Check sheet for the modelled part. Datum: model origin and axes. Units: mm. A direction names the side the tool comes from. Coordinates: 2 decimals unless noted, no trailing zeros. Loops run counter-clockwise (first coordinate to the right, second up) from the corner with the lowest first, then second, coordinate; pieces in that order, holes last. Notation, with made-up numbers: (-23.5, 71) -> (34.5, 71) arc R25 cw to (34.5, 96) -> close; hole circle Ø7 at (-35, 41.25). An arc over 180 degrees is marked (long way). Use CSV: the item, a comma, the result in double quotes.
```python
from build123d import *

# Parameters (mm, degrees)
SKETCH1_W                      = 105
SKETCH1_H                      = 69
BOSS_EXTRUDE1_DEPTH            = 10
FILLET1_R                      = 3
CBORE_FOR_M3_SHCS1_D           = 3.4
CBORE_FOR_M3_SHCS1_CBORE_D     = 6.5
CBORE_FOR_M3_SHCS1_CBORE_DEPTH = 4


with BuildPart() as part:
    # Sketch1 → Boss-Extrude1 (new body)
    with BuildSketch(Plane(origin=(0, 0, 0), x_dir=(1, 0, 0), z_dir=(0, 1, 0))):
        Rectangle(SKETCH1_W, SKETCH1_H)
    extrude(amount=BOSS_EXTRUDE1_DEPTH)

    # Fillet1
    fillet1_edges = [part.edges().sort_by_distance(p)[0] for p in [
        (52.5, 5, 34.5),
        (-52.5, 5, 34.5),
        (-52.5, 5, -34.5),
        (52.5, 5, -34.5),
    ]]
    fillet(fillet1_edges, radius=FILLET1_R)

    # CBORE for M3 SHCS1 (through all)
    with Locations(Plane(origin=(0, 10, 0), x_dir=(1, 0, 0), z_dir=(0, 1, 0))):
        with Locations((0, 0)):
            CounterBoreHole(CBORE_FOR_M3_SHCS1_D / 2, CBORE_FOR_M3_SHCS1_CBORE_D / 2, CBORE_FOR_M3_SHCS1_CBORE_DEPTH)

    # Sketch5 → M3x0.5 Tapped Hole1 (revolve, cut)
    with BuildSketch(Plane(origin=(16.5, 10, 22), x_dir=(0, 0, 1), z_dir=(1, 0, 0))):
        Polygon((0, 0), (0, 10.751075774), (1.25, 10), (1.25, 0), align=None)
    m3x0_5_tapped_hole1 = revolve(axis=Axis((16.5, 16.35, 22), (0, -1, 0)), mode=Mode.SUBTRACT)

    # Mirror1: M3x0.5 Tapped Hole1 across plane
    add(m3x0_5_tapped_hole1.mirror(Plane(origin=(0, 0, 0), x_dir=(0, 0, 1), z_dir=(1, 0, 0))), mode=Mode.SUBTRACT)

    # Mirror2: M3x0.5 Tapped Hole1 across plane
    add(m3x0_5_tapped_hole1.mirror(Plane.XY), mode=Mode.SUBTRACT)

    # Mirror2 copy 1 sketch → Mirror2 copy 1 (revolve, cut)
    with BuildSketch(Plane(origin=(-16.5, 10, -22), x_dir=(0, 0, -1), z_dir=(-1, 0, 0))):
        Polygon((0, 0), (0, 10.751075774), (1.25, 10), (1.25, 0), align=None)
    revolve(axis=Axis((-16.5, 16.35, -22), (0, -1, 0)), mode=Mode.SUBTRACT)


solid = part.part
```
1) Cross-section at C-C on z = -22. Record the boundary of the cut face in (x, y), and give its area (3 significant figures).
Answer below:
outline,"(-52.5, 0) -> (-17.75, 0) -> (-17.75, 10) -> (-52.5, 10) -> close; (-15.25, 0) -> (15.25, 0) -> (15.25, 10) -> (-15.25, 10) -> close; (17.75, 0) -> (52.5, 0) -> (52.5, 10) -> (17.75, 10) -> close"
area,"1,000 mm²"
2) Draft check along Z on faces 3 (the flat face through (-1, 5, 34.5)), 4 (the flat face through (52.5, 5, 0)), 5 (the cylindrical face through (-2.579, 8.028, 1.978)). Enter one of: released by +Z, released by -Z, zero draft, split by the parting line, or undercut.
Answer below:
face 3,"released by +Z"
face 4,"zero draft"
face 5,"undercut"
3) Cross-section at A-A on z = 0. Record the boundary of the cut face in (x, y), and give its area (3 significant figures).
Answer below:
outline,"(-52.5, 0) -> (-1.7, 0) -> (-1.7, 6) -> (-3.25, 6) -> (-3.25, 10) -> (-52.5, 10) -> close; (1.7, 0) -> (52.5, 0) -> (52.5, 10) -> (3.25, 10) -> (3.25, 6) -> (1.7, 6) -> close"
area,"1,000 mm²"
4) Cross-section at B-B on x = 0. Record the boundary of the cut face in (y, z), and give its area (3 significant figures).
Answer below:
outline,"(0, -34.5) -> (10, -34.5) -> (10, -3.25) -> (6, -3.25) -> (6, -1.7) -> (0, -1.7) -> close; (0, 1.7) -> (6, 1.7) -> (6, 3.25) -> (10, 3.25) -> (10, 34.5) -> (0, 34.5) -> close"
area,"644 mm²"
5) Thickness scan on line 1 along X through (y, z) = (3.75, -22); line 2 along Z through (x, y) = (16.5, 4.25); line 3 along Z through (x, y) = (0, 4.75). Record the ranges inside material, lowest first. Write a range as from..to.
Answer below:
line 1,"x = -52.5..-17.75, -15.25..15.25, 17.75..52.5"
line 2,"z = -34.5..-23.25, -20.75..20.75, 23.25..34.5"
line 3,"z = -34.5..-1.7, 1.7..34.5"
6) Go/stop test with flat-tipped pins: pin 1 Ø4 at (x, z) = (-16.5, 22) entering from +Y; pin 2 Ø4.5 at (x, z) = (0, 0) entering from +Y. Record where each tip stops, or that it passes through.
Answer below:
pin 1,"stops at y = 10"
pin 2,"stops at y = 6"
7) Access from +Z, -Z, +X, -X, +Y, -Y to the whole of each face (thin tool, end or side, straight path). Record for faces 1 (the flat face through (1.4, 6, 1.4)), 2 (the cylindrical face through (15.446, 5.07, -22.672)).
Answer below:
face 1,"+Y"
face 2,"+Y, -Y"
8) Cross-section at D-D on x = -16.5. Record the boundary of the cut face in (y, z).
Answer below:
outline,"(0, -34.5) -> (10, -34.5) -> (10, -23.25) -> (0, -23.25) -> close; (0, -20.75) -> (10, -20.75) -> (10, 20.75) -> (0, 20.75) -> close; (0, 23.25) -> (10, 23.25) -> (10, 34.5) -> (0, 34.5) -> close"
